Verification items for the finished model (mm, model axes). A direction names the side the tool comes from. Give positions to 0.01 mm unless a question says otherwise; leave off trailing zeros. Write each loop counter-clockwise with the first axis right and the second up, starting at its lowest first coordinate (ties: lowest second). Pieces come first, ordered by that corner, then holes. Notation, with made-up numbers: (21, -25.5) -> (33, -25.5) arc R33 cw to (33, 3.5) -> close; hole circle Ø2 at (37.25, -24). An arc over 180 degrees is marked (long way). Answer as CSV lines item,"result".
```python
from build123d import *

# Parameters (mm, degrees)
BOSS_EXTRUDE1_DEPTH = 65.8876
BOSS_EXTRUDE2_DEPTH = 29.3624
SKETCH4_R           = 2
BOSS_EXTRUDE3_DEPTH = 13.8684
FILLET1_R           = 1.27


with BuildPart() as part:
    # Sketch1 → Boss-Extrude1 (new body)
    with BuildSketch(Plane(origin=(0, 0, 0), x_dir=(1, 0, 0), z_dir=(0, 1, 0))):
        with BuildLine():
            Line((-12.2809, 0), (-15.4559, 0))
            Line((-15.4559, 0), (-15.4559, -13.3604))
            Line((-15.4559, -13.3604), (-15.4559, -13.8684))
            Line((-15.4559, -13.8684), (0, -13.8684))
            Line((0, -13.8684), (15.4559, -13.8684))
            Line((15.4559, -13.8684), (15.4559, -13.3604))
            Line((15.4559, -13.3604), (15.4559, 0))
            Line((15.4559, 0), (12.2809, 0))
            ThreePointArc((12.2809, 0), (0, -12.2809), (-12.2809, 0))
        make_face()
    extrude(amount=BOSS_EXTRUDE1_DEPTH)

    # Sketch2 → Boss-Extrude2 (add)
    with BuildSketch(Plane(origin=(0, 65.8876, 0), x_dir=(1, 0, 0), z_dir=(0, 1, 0))):
        Polygon((-12.2809, -12.2809), (0, -12.2809), (12.2809, -12.2809), (15.4559, -12.2809), (15.4559, -13.3604), (15.4559, -13.8684), (-15.4559, -13.8684), (-15.4559, -13.3604), (-15.4559, -12.2809), align=None)
    boss_extrude2 = extrude(amount=BOSS_EXTRUDE2_DEPTH)

    # Mirror1: Boss-Extrude2 across plane
    add(boss_extrude2.mirror(Plane.ZX.offset(32.9438)))

    # Sketch4 → Boss-Extrude3 (add, through all)
    # profile 1 of 6: a face of its own
    with BuildSketch(Plane(origin=(0, 0, 0), x_dir=(-1, 0, 0), z_dir=(0, 0, -1))):
        with BuildLine():
            Line((-15.4559, 39.2938), (-15.4559, 26.5938))
            Line((-15.4559, 26.5938), (-18.6309, 26.5938))
            ThreePointArc((-18.6309, 26.5938), (-24.9809, 32.9438), (-18.6309, 39.2938))
            Line((-18.6309, 39.2938), (-15.4559, 39.2938))
        make_face()
        with Locations((-18.6309, 32.9438)):
            Circle(SKETCH4_R, mode=Mode.SUBTRACT)
    # profile 2 of 6: a face of its own
    with BuildSketch(Plane(origin=(0, 0, 0), x_dir=(-1, 0, 0), z_dir=(0, 0, -1))):
        with BuildLine():
            Line((-15.4559, 12.7), (-18.6309, 12.7))
            ThreePointArc((-18.6309, 12.7), (-24.9809, 6.35), (-18.6309, 0))
            Line((-18.6309, 0), (-15.4559, 0))
            Line((-15.4559, 0), (-15.4559, 12.7))
        make_face()
        with Locations(Location((-18.6309, 6.35, 0), (0, 0, 180))):
            Circle(SKETCH4_R, mode=Mode.SUBTRACT)
    # profile 3 of 6: a face of its own
    with BuildSketch(Plane(origin=(0, 0, 0), x_dir=(-1, 0, 0), z_dir=(0, 0, -1))):
        with BuildLine():
            Line((-18.6309, 65.8876), (-15.4559, 65.8876))
            Line((-15.4559, 65.8876), (-15.4559, 53.1876))
            Line((-15.4559, 53.1876), (-18.6309, 53.1876))
            ThreePointArc((-18.6309, 53.1876), (-24.9809, 59.5376), (-18.6309, 65.8876))
        make_face()
        with Locations((-18.6309, 59.5376)):
            Circle(SKETCH4_R, mode=Mode.SUBTRACT)
    # profile 4 of 6: a face of its own
    with BuildSketch(Plane(origin=(0, 0, 0), x_dir=(-1, 0, 0), z_dir=(0, 0, -1))):
        with BuildLine():
            Line((18.6309, 0), (15.4559, 0))
            Line((15.4559, 0), (15.4559, 12.7))
            Line((15.4559, 12.7), (18.6309, 12.7))
            ThreePointArc((18.6309, 12.7), (24.9809, 6.35), (18.6309, 0))
        make_face()
        with Locations((18.6309, 6.35)):
            Circle(SKETCH4_R, mode=Mode.SUBTRACT)
    # profile 5 of 6: a face of its own
    with BuildSketch(Plane(origin=(0, 0, 0), x_dir=(-1, 0, 0), z_dir=(0, 0, -1))):
        with BuildLine():
            Line((15.4559, 53.1876), (18.6309, 53.1876))
            ThreePointArc((18.6309, 53.1876), (24.9809, 59.5376), (18.6309, 65.8876))
            Line((18.6309, 65.8876), (15.4559, 65.8876))
            Line((15.4559, 65.8876), (15.4559, 53.1876))
        make_face()
        with Locations(Location((18.6309, 59.5376, 0), (0, 0, 180))):
            Circle(SKETCH4_R, mode=Mode.SUBTRACT)
    # profile 6 of 6: a face of its own
    with BuildSketch(Plane(origin=(0, 0, 0), x_dir=(-1, 0, 0), z_dir=(0, 0, -1))):
        with BuildLine():
            Line((18.6309, 26.5938), (15.4559, 26.5938))
            Line((15.4559, 26.5938), (15.4559, 39.2938))
            Line((15.4559, 39.2938), (18.6309, 39.2938))
            ThreePointArc((18.6309, 39.2938), (24.9809, 32.9438), (18.6309, 26.5938))
        make_face()
        with Locations(Location((18.6309, 32.9438, 0), (0, 0, 180))):
            Circle(SKETCH4_R, mode=Mode.SUBTRACT)
    extrude(amount=-BOSS_EXTRUDE3_DEPTH)

    # Fillet1
    fillet1_edges = [part.edges().sort_by_distance(p)[0] for p in [
        (-15.4559, 65.8876, 13.07465),
        (-15.4559, 0, 13.07465),
        (15.4559, 95.25, 13.07465),
        (-15.4559, 95.25, 13.07465),
        (-15.4559, -29.3624, 13.07465),
        (15.4559, -29.3624, 13.07465),
        (15.4559, 65.8876, 13.07465),
        (15.4559, 0, 13.07465),
    ]]
    fillet(fillet1_edges, radius=FILLET1_R)


solid = part.part
```
1) Section check C-C (x = -5). Record the boundary of the cut face in (y, z).
Reported:
outline,"(-29.36, 12.28) -> (0, 12.28) -> (0, 11.22) -> (65.89, 11.22) -> (65.89, 12.28) -> (95.25, 12.28) -> (95.25, 13.87) -> (-29.36, 13.87) -> close"
2) Section check A-A (z = 5). State how many separate pieces and enclosed holes the cut face has, and give its area (3 significant figures).
Reported:
separate pieces,"2"
enclosed holes,"6"
area,"1,110 mm²"
3) Tool access check on faces 1 (the flat face through (17, 26.594, 7)), 2 (the flat face through (16, 33, 0)), 3 (the flat face through (-17, 39.294, 7)). Record the directions out of +Z, -Z, +X, -X, +Y, -Y that give a thin tool (end or side, any length) a straight path to the whole face; none if there is none.
Reported:
face 1,"+Z, -Z, +X"
face 2,"-Z, +X, -X, +Y, -Y"
face 3,"+Z, -Z, -X"
4) Scan lines: line 1 along Y through (x, z) = (-18, 10); line 2 along X through (y, z) = (34.5, 2.25); line 3 along Y through (x, z) = (17, 2). Record each from-to range of solid material in increasing order.
Reported:
line 1,"0 to 4.45, 8.25 to 12.7, 26.59 to 31.05, 34.84 to 39.29, 53.19 to 57.64, 61.44 to 65.89"
line 2,"-24.79 to -19.89, -17.37 to -12.07, 12.07 to 17.37, 19.89 to 24.79"
line 3,"0 to 5.19, 7.51 to 12.7, 26.59 to 31.79, 34.1 to 39.29, 53.19 to 58.38, 60.7 to 65.89"
5) Section check B-B (y = 6.35). Record the boundary of the cut face in (x, z).
Reported:
outline,"(-24.98, 0) -> (-20.63, 0) -> (-20.63, 13.87) -> (-24.98, 13.87) -> close; (-16.63, 0) -> (-12.28, 0) arc R12.28 cw to (12.28, 0) -> (16.63, 0) -> (16.63, 13.87) -> (-16.63, 13.87) -> close; (20.63, 0) -> (24.98, 0) -> (24.98, 13.87) -> (20.63, 13.87) -> close"
6) Depth check by flat-ended pin: pin 1 (1.7 mm diameter, centred on y = 75.5, z = 12.5, fed in from -X); pin 2 (0.5 mm diameter, centred on y = -18, z = 12.5, fed in from +X); pin 3 (2.5 mm diameter, centred on x = 16.5, z = 4, fed in from -Y). Enter the tip coordinate at first touch or a pass-through.
Reported:
pin 1,"x = -15.46"
pin 2,"x = 15.46"
pin 3,"y = 0"
7) Draft check along Y on faces 4 (the cylindrical face through (-24.98, 6.49, 6.84)), 5 (the flat face through (0, 80, 12.281)), 6 (the flat face through (14, 0, 7)). Enter one of: +Y half, -Y half, draft (parallel to the pull), parting line (faces both ways), or undercut.
Reported:
face 4,"undercut"
face 5,"draft"
face 6,"-Y half"
8) Section check D-D (y = 24). Record the boundary of the cut face in (x, z).
Reported:
outline,"(-15.46, 0) -> (-12.28, 0) arc R12.28 cw to (12.28, 0) -> (15.46, 0) -> (15.46, 13.87) -> (-15.46, 13.87) -> close"
